Design review of the part built by this model. Coordinates are the model's own, in mm. A direction names the side the tool comes from. Coordinates: 2 decimals unless noted, no trailing zeros. Order: outer loops, then holes, each group sorted by start corner. A loop starts at its lowest first (then second) coordinate and runs counter-clockwise, first axis right, second up.
from build123d import *

# Parameters (mm, degrees)
F0_W     = 40
F0_H     = 40
F0_R     = 1.75
F0_R_2   = 19.1
F1_DEPTH = 14
F3_DEPTH = 10
F4_R     = 2.5
F6_DEPTH = 4


with BuildPart() as f1:
    # F0 (on Front) → F1 (new body, symmetric)
    with BuildSketch(Plane.XZ):
        Rectangle(F0_W, F0_H)
        with Locations((-16, -16)):
            Circle(F0_R, mode=Mode.SUBTRACT)
        with Locations((16, -16)):
            Circle(F0_R, mode=Mode.SUBTRACT)
        with Locations((-16, 16)):
            Circle(F0_R, mode=Mode.SUBTRACT)
        Circle(F0_R_2, mode=Mode.SUBTRACT)
        with Locations((16, 16)):
            Circle(F0_R, mode=Mode.SUBTRACT)
    extrude(amount=F1_DEPTH, both=True)

    # F2 (on Front) → F3 (cut, symmetric)
    with BuildSketch(Plane.XZ):
        with BuildLine():
            ThreePointArc((-15.8567471072, 12.8282333616), (-18.2450640303, 18.2450640303), (-12.8282333616, 15.8567471072))
            ThreePointArc((-12.8282333616, 15.8567471072), (-8.6653906808, 18.463775463), (-4, 20))
            Line((-4, 20), (-4, 20.3960780544))
            Line((-4, 20.3960780544), (-20.3960780544, 20.3960780544))
            Line((-20.3960780544, 20.3960780544), (-20.3960780544, 4))
            Line((-20.3960780544, 4), (-20, 4))
            ThreePointArc((-20, 4), (-18.463775463, 8.6653906808), (-15.8567471072, 12.8282333616))
        make_face()
        with BuildLine():
            Line((20.3960780544, 4), (20.3960780544, 20.3960780544))
            Line((20.3960780544, 20.3960780544), (4, 20.3960780544))
            Line((4, 20.3960780544), (4, 20))
            ThreePointArc((4, 20), (8.6653906808, 18.463775463), (12.8282333616, 15.8567471072))
            ThreePointArc((12.8282333616, 15.8567471072), (18.2450640303, 18.2450640303), (15.8567471072, 12.8282333616))
            ThreePointArc((15.8567471072, 12.8282333616), (18.463775463, 8.6653906808), (20, 4))
            Line((20, 4), (20.3960780544, 4))
        make_face()
        with BuildLine():
            Line((-20.3960780544, -4), (-20.3960780544, -20.3960780544))
            Line((-20.3960780544, -20.3960780544), (-4, -20.3960780544))
            Line((-4, -20.3960780544), (-4, -20))
            ThreePointArc((-4, -20), (-8.6653906808, -18.463775463), (-12.8282333616, -15.8567471072))
            ThreePointArc((-12.8282333616, -15.8567471072), (-18.2450640303, -18.2450640303), (-15.8567471072, -12.8282333616))
            ThreePointArc((-15.8567471072, -12.8282333616), (-18.463775463, -8.6653906808), (-20, -4))
            Line((-20, -4), (-20.3960780544, -4))
        make_face()
        with BuildLine():
            Line((4, -20.3960780544), (20.3960780544, -20.3960780544))
            Line((20.3960780544, -20.3960780544), (20.3960780544, -4))
            Line((20.3960780544, -4), (20, -4))
            ThreePointArc((20, -4), (18.463775463, -8.6653906808), (15.8567471072, -12.8282333616))
            ThreePointArc((15.8567471072, -12.8282333616), (18.2450640303, -18.2450640303), (12.8282333616, -15.8567471072))
            ThreePointArc((12.8282333616, -15.8567471072), (8.6653906808, -18.463775463), (4, -20))
            Line((4, -20), (4, -20.3960780544))
        make_face()
    extrude(amount=F3_DEPTH, both=True, mode=Mode.SUBTRACT)

    # F4
    f4_edges = [f1.edges().sort_by_distance(p)[0] for p in [
        (20, -12, 20),
        (20, 12, 20),
        (20, -12, -20),
        (20, 12, -20),
        (-20, -12, 20),
        (-20, 12, 20),
        (-20, 12, -20),
        (-20, -12, -20),
    ]]
    fillet(f4_edges, radius=F4_R)

    # F5 (on face) → F6 (join)
    with BuildSketch(Plane.XZ.offset(14)):
        with BuildLine():
            Line((-3.6, 18.7576650999), (-3.6, 12.1790804251))
            ThreePointArc((-3.6, 12.1790804251), (-11.5533772944, 5.2734687913), (-11.5597385217, -5.2595099877))
            Line((-11.5597385217, -5.2595099877), (-17.1195297525, -8.4694569515))
            ThreePointArc((-17.1195297525, -8.4694569515), (-16.5410852123, -9.55), (-15.8945297525, -10.5912191908))
            Line((-15.8945297525, -10.5912191908), (-10.3347385217, -7.381272227))
            ThreePointArc((-10.3347385217, -7.381272227), (0, -12.7), (10.3347385217, -7.381272227))
            Line((10.3347385217, -7.381272227), (15.8945297525, -10.5912191908))
            ThreePointArc((15.8945297525, -10.5912191908), (16.5410852123, -9.55), (17.1195297525, -8.4694569515))
            Line((17.1195297525, -8.4694569515), (11.5597385217, -5.2595099877))
            ThreePointArc((11.5597385217, -5.2595099877), (11.5533772944, 5.2734687913), (3.6, 12.1790804251))
            Line((3.6, 12.1790804251), (3.6, 18.7576650999))
            ThreePointArc((3.6, 18.7576650999), (0, 19.1), (-3.6, 18.7576650999))
        make_face()
    extrude(amount=-F6_DEPTH)

    # F7 (on Right) → F8 (revolve)
    with BuildSketch(Plane.YZ):
        Polygon((-10, 0), (14, 0), (14, 7.5), (4, 12.7), (-10, 12.7), align=None)
    revolve(axis=Axis((0, 1.2222109362, 0), (0, 1, 0)))


solid = f1.part
1. Add section B-B (x = 0). Give the boundary of the cut face in (y, z).
2. For faces 5 (the cylindrical face through (-18.32, 0.14, 18.17)), 6 (the flat face through (-14, -10, -8)), 7 (the flat face through (0, 0, -20)), 8 (the flat face through (3.6, -12, 15)), list the 3-axis set-ups (+Z, -Z, +X, -X, +Y, -Y) from which the entire face can be reached by the end or side of a thin tool; tool diameter is ignored.
3. Mouldability with a two-part tool opening along Y and no side actions: class faces 1 (the flat face through (13.076, -12.028, -8.964)), 2 (the flat face through (12.6, 10, -16.7)), 3 (the flat face through (0, -10, 16)), 4 (the flat face through (16.7, 10, 12.6)) as pulls with the +Y half, pulls with the -Y half, needs draft (parallel to the pull), parting line crosses it, or undercut.
4. Add section D-D (y = 1.5). Give the boundary of the cut face in (x, z) (3 decimals), and give its area (3 significant figures).
5. Add section C-C (z = 0). Give the boundary of the cut face in (x, y).
6. To check wall thickness, follow line 1 (X direction, y = -4, z = 0.5); line 2 (Z direction, x = -16, y = 3) (3 decimals); line 3 (Z direction, x = 0, y = 9). State the ranges of each line that lie inside material, in increasing order.
7. Add section A-A (y = 10.75). Give the boundary of the cut face in (x, z), and give its area (3 significant figures).
8. Insertion check: pin 1 (2.5 mm diameter, centred on x = -12.5, z = -8.5, fed in from +Y); pin 2 (4 mm diameter, centred on y = -1.5, z = -12.5, fed in from +X); pin 3 (5 mm diameter, centred on y = -3.5, z = 15.5, fed in from -X) (3 decimals). Each pin has a flat end and moves straight along its axis. Give the tip position at first contact, or say it passes through.
Solution:
1. outline: (-14, -20) - (14, -20) - (14, -19.1) - (-14, -19.1) - close; (-14, -12.7) - (4, -12.7) - (14, -7.5) - (14, 7.5) - (4, 12.7) - (-10, 12.7) - (-10, 19.1) - (14, 19.1) - (14, 20) - (-14, 20) - close
2. face 5: none
2. face 6: +Y
2. face 7: -Z, +X, -X, +Y, -Y
2. face 8: +Y, -Y
3. face 1: needs draft
3. face 2: undercut
3. face 3: pulls with the +Y half
3. face 4: undercut
4. outline: (-20, -4) arc R20.396 ccw to (-15.857, -12.828) arc R3.175 ccw (long way) to (-12.828, -15.857) arc R20.396 ccw to (-4, -20) - (4, -20) arc R20.396 ccw to (12.828, -15.857) arc R3.175 ccw (long way) to (15.857, -12.828) arc R20.396 ccw to (20, -4) - (20, 4) arc R20.396 ccw to (15.857, 12.828) arc R3.175 ccw (long way) to (12.828, 15.857) arc R20.396 ccw to (4, 20) - (-4, 20) arc R20.396 ccw to (-12.828, 15.857) arc R3.175 ccw (long way) to (-15.857, 12.828) arc R20.396 ccw to (-20, 4) - close; circle Ø25.4 at (0, 0); hole circle Ø38.2 at (0, 0); hole circle Ø3.5 at (-16, -16); hole circle Ø3.5 at (-16, 16); hole circle Ø3.5 at (16, -16); hole circle Ø3.5 at (16, 16)
4. area: 736 mm2
5. outline: (-20, -14) - (-19.1, -14) - (-19.1, 14) - (-20, 14) - close; (-12.7, -14) - (12.7, -14) - (12.7, 4) - (7.5, 14) - (-7.5, 14) - (-12.7, 4) - close; (19.1, -14) - (20, -14) - (20, 14) - (19.1, 14) - close
6. line 1: x = -20 to -19.09, -12.69 to 12.69, 19.09 to 20
6. line 2: z = -19.175 to -17.75, -14.25 to -12.825, -12.649 to -10.431, 10.431 to 12.649, 12.825 to 14.25, 17.75 to 19.175
6. line 3: z = -20 to -19.1, -10.1 to 10.1, 19.1 to 20
7. outline: (-20, -17.5) arc R2.5 ccw to (-17.5, -20) - (17.5, -20) arc R2.5 ccw to (20, -17.5) - (20, 17.5) arc R2.5 ccw to (17.5, 20) - (-17.5, 20) arc R2.5 ccw to (-20, 17.5) - close; circle Ø18.38 at (0, 0); hole circle Ø38.2 at (0, 0); hole circle Ø3.5 at (-16, -16); hole circle Ø3.5 at (-16, 16); hole circle Ø3.5 at (16, -16); hole circle Ø3.5 at (16, 16)
7. area: 675 mm2
8. pin 1: stops at y = -10
8. pin 2: stops at x = 18.8
8. pin 3: stops at x = -19.175
